Print and shaded views of the part. All mm, measured from the part's lowest x, y and z. Give positions to 0.01 mm unless a question says otherwise; leave off trailing zeros. Loops run counter-clockwise (first coordinate to the right, second up) from the corner with the lowest first, then second, coordinate; pieces in that order, holes last. Notation, with made-up numbers: (66, 59.25) -> (73, 59.25) arc R25 cw to (73, 95.25) -> close; hole circle Ø4 at (54, -21.5). An arc over 180 degrees is marked (long way). Answer as a JSON object with one key per item and string values. Group by question number.
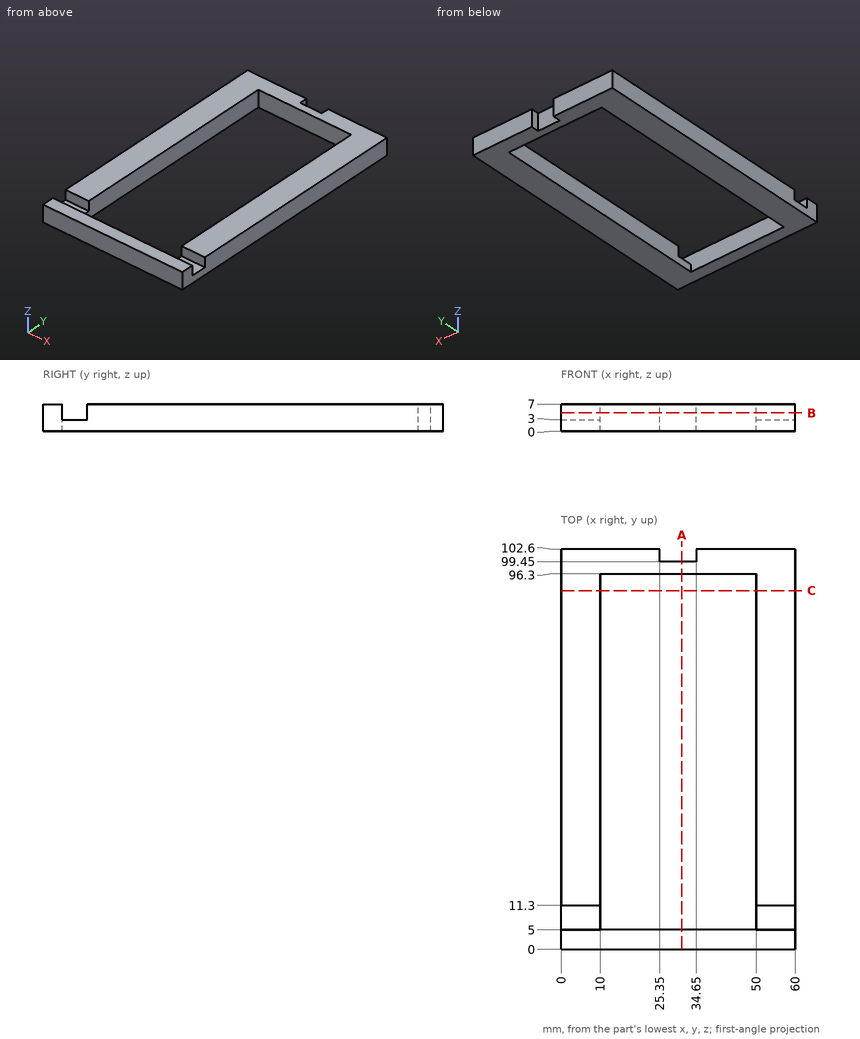
(1) Saw through at C-C on y = 92. List the corners of the cut face in (x, z), plus the area to 3 significant figures.
(2) Pin check, flat tips, straight feed: pin 1 (12 mm diameter, centred on x = 42.5, y = 28.5, fed in from +Z); pin 2 (3 mm diameter, centred on x = 3, y = 7.5, fed in from +Z). Stop position of each tip, or through.
(3) Saw through at B-B on z = 4.75. List the corners of the cut face in (x, y), plus the area to 3 significant figures.
(4) Saw through at A-A on x = 31. List the corners of the cut face in (y, z), plus the area to 4 significant figures.
(5) Probe line 1 along X through (y, z) = (84, 3.25); line 2 along Y through (x, z) = (35, 2); line 3 along Y through (x, z) = (29, 1.25). List the from-to ranges inside material, lowest first. Write a range as [from, to].
Calculated:
{
 "1": {"outline": "(0, 0) -> (10, 0) -> (10, 7) -> (0, 7) -> close; (50, 0) -> (60, 0) -> (60, 7) -> (50, 7) -> close", "area": "140 mm^2"},
 "2": {"pin 1": "passes through", "pin 2": "stops at z = 3"},
 "3": {"outline": "(0, 0) -> (60, 0) -> (60, 5) -> (0, 5) -> close; (0, 11.3) -> (10, 11.3) -> (10, 96.3) -> (50, 96.3) -> (50, 11.3) -> (60, 11.3) -> (60, 102.6) -> (34.65, 102.6) -> (34.65, 99.45) -> (25.35, 99.45) -> (25.35, 102.6) -> (0, 102.6) -> close", "area": "2,350 mm^2"},
 "4": {"outline": "(0, 0) -> (5, 0) -> (5, 7) -> (0, 7) -> close; (96.3, 0) -> (99.45, 0) -> (99.45, 7) -> (96.3, 7) -> close", "area": "57.05 mm^2"},
 "5": {"line 1": "x = [0, 10], [50, 60]", "line 2": "y = [0, 5], [96.3, 102.6]", "line 3": "y = [0, 5], [96.3, 99.45]"}
}
